Can you work these out from the model? Positions are in its coordinate system, mm. Face numbers are marked on the shaded views. A direction names the side the tool comes from. Coordinates: 2 decimals unless noted, no trailing zeros. Order: outer loops, then holes, each group sorted by start corner. A loop starts at its lowest first (then second) coordinate and runs counter-clockwise, first axis right, second up. Notation, with made-up numbers: M 30.5,9.25 L 52.5,9.25 A28 cw 52.5,44.25 Z; hole C 75,72 d2. An arc over 180 degrees is marked long. Answer as a JSON object with one key per item and string values.
from build123d import *
from build123d import SkipClean  # not in build123d's __all__

# Parameters (mm, degrees)
F1_DEPTH = 31.75
F2_DEPTH = 53.975
F3_DEPTH = 73.025
F0_W     = 31.75
F0_H     = 31.75
F4_DEPTH = 92.075
F5_DEPTH = 73.025


with BuildPart() as f1:
    # F0 (on Top) → F1 (new body)
    with BuildSketch(Plane.XY):
        Polygon((108.4912913322, 117.0880892358), (32.2912913322, 117.0880892358), (32.2912913322, 85.3380892358), (32.2912913322, 15.4880892358), (32.2912913322, -3.5619107642), (32.2912913322, -16.2619107642), (32.2912913322, -35.3119107642), (108.4912913322, -35.3119107642), (108.4912913322, 15.4880892358), (67.2162913322, 15.4880892358), (67.2162913322, 66.2880892358), (108.4912913322, 66.2880892358), align=None)
    extrude(amount=F1_DEPTH)



with BuildPart() as f2:
    # F0 (on Top) → F2 (new body)
    with BuildSketch(Plane.XY):
        with BuildLine():
            Line((0.5412913322, 117.0880892358), (-37.5587086678, 117.0880892358))
            Line((-37.5587086678, 117.0880892358), (-37.5587086678, 56.7630892358))
            ThreePointArc((-37.5587086678, 56.7630892358), (-21.6837086678, 40.8880892358), (-37.5587086678, 25.0130892358))
            Line((-37.5587086678, 25.0130892358), (-37.5587086678, -35.3119107642))
            Line((-37.5587086678, -35.3119107642), (0.5412913322, -35.3119107642))
            Line((0.5412913322, -35.3119107642), (0.5412913322, -3.5619107642))
            Line((0.5412913322, -3.5619107642), (0.5412913322, 15.4880892358))
            Line((0.5412913322, 15.4880892358), (0.5412913322, 85.3380892358))
            Line((0.5412913322, 85.3380892358), (0.5412913322, 117.0880892358))
        make_face()
    extrude(amount=F2_DEPTH)


with BuildPart() as f1_1:
    add(f1.part, clean=False)

    add(f2.part)  # F3 merges F2
    # F0 (on Top) → F3 (join)
    with BuildSketch(Plane.XY):
        Polygon((32.2912913322, 85.3380892358), (0.5412913322, 85.3380892358), (0.5412913322, 15.4880892358), (0.5412913322, -3.5619107642), (32.2912913322, -3.5619107642), (32.2912913322, 15.4880892358), align=None)
    extrude(amount=F3_DEPTH)

    # F0 (on Top) → F4 (join)
    with BuildSketch(Plane.XY):
        Polygon((32.2912913322, -3.5619107642), (0.5412913322, -3.5619107642), (0.5412913322, -35.3119107642), (32.2912913322, -35.3119107642), (32.2912913322, -16.2619107642), align=None)
        with Locations((16.4162913322, 101.2130892358)):
            Rectangle(F0_W, F0_H)
    extrude(amount=F4_DEPTH)

    # F0 (on Top) → F5 (join)
    with BuildSketch(Plane.XY):
        Polygon((32.2912913322, 85.3380892358), (0.5412913322, 85.3380892358), (0.5412913322, 15.4880892358), (0.5412913322, -3.5619107642), (32.2912913322, -3.5619107642), (32.2912913322, 15.4880892358), align=None)
    extrude(amount=F5_DEPTH)

    # F6: F1 across face


with BuildPart() as f1_2:
    add(f1_1.part, clean=False)
    with SkipClean():  # cleaning this boolean's faces spoils the solid; the shape is the same uncleaned
        add(f1_1.part.mirror(Plane(origin=(-37.5587086678, 86.9255892358, 26.9875), x_dir=(0, -1, 0), z_dir=(-1, 0, 0))), clean=False)


solid = f1_2.part
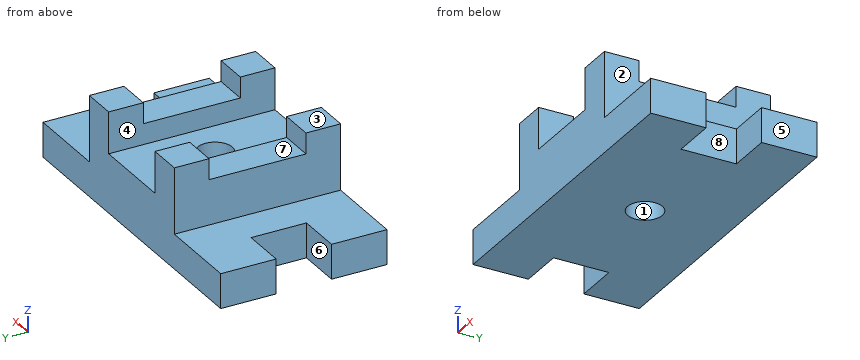
Item 1: I want a section at A-A, the plane x = 74. Write out the boundary of the cut face in (y, z), plus the area to 3 significant figures.
Answers follow:
{"outline": "M -35.31,0 L 15.49,0 L 15.49,31.75 L -35.31,31.75 Z; M 66.29,0 L 117.09,0 L 117.09,31.75 L 66.29,31.75 Z", "area": "3,230 mm^2"}
Item 2: I want a section at D-D, the plane x = 21. Write out the boundary of the cut face in (y, z) (3 decimals).
Answers follow:
{"outline": "M -35.312,0 L 117.088,0 L 117.088,92.075 L 85.338,92.075 L 85.338,73.025 L -3.562,73.025 L -3.562,92.075 L -35.312,92.075 Z"}
Item 3: Please list where these lines run through material, in increasing order: line 1 (X direction, y = -5, z = 70.5); line 2 (Y direction, x = 93, z = 12); line 3 (Y direction, x = -100, z = 74).
Answers follow:
{"line 1": "x = -107.41 to -75.66, 0.54 to 32.29", "line 2": "y = -35.31 to 15.49, 66.29 to 117.09", "line 3": "y = -35.31 to -3.56, 85.34 to 117.09"}
Item 4: If we mould it in two halves opening along X, with no side actions, what happens to the marked faces 1, 2 and 3? For each: pulls with the +X half, pulls with the -X half, needs draft (parallel to the pull), parting line crosses it, or undercut.
Answers follow:
{"face 1": "undercut", "face 2": "pulls with the +X half", "face 3": "needs draft"}
Item 5: Which directions (+Z, -Z, +X, -X, +Y, -Y) give clear straight access to the entire face, cutting with the end or side of a thin tool? Please do the marked faces 4, 5, 6, 7 and 8.
Answers follow:
{"face 4": "+Z, +Y, -Y", "face 5": "+Z, -Z, +X, +Y, -Y", "face 6": "+Z, -Z, -X", "face 7": "+Z, +X, -X", "face 8": "+Z, -Z, +X"}
Item 6: I want a section at C-C, the plane y = -7. Write out the boundary of the cut face in (x, z) (3 decimals), plus the area to 3 significant figures.
Answers follow:
{"outline": "M -183.609,0 L 108.491,0 L 108.491,31.75 L 32.291,31.75 L 32.291,92.075 L 0.541,92.075 L 0.541,53.975 L -75.659,53.975 L -75.659,92.075 L -107.409,92.075 L -107.409,31.75 L -183.609,31.75 Z", "area": "14,800 mm^2"}
Item 7: I'm going to push flat-ended pins straight in: pin 1 (19 mm diameter, centred on x = -37.56, y = 40.89, fed in from -Z); pin 2 (6 mm diameter, centred on y = 13, z = 57, fed in from +X); pin 3 (4 mm diameter, centred on x = -34, y = 9, fed in from -Z); pin 4 (12 mm diameter, centred on y = 55, z = 28.5, fed in from +X). Where does each tip first touch, or does it pass through?
Answers follow:
{"pin 1": "passes through", "pin 2": "stops at x = 32.29", "pin 3": "stops at z = 0", "pin 4": "stops at x = 67.22"}
Item 8: I want a section at B-B, the plane z = 69. Write out the boundary of the cut face in (x, y), plus the area to 3 significant figures.
Answers follow:
{"outline": "M -107.41,-35.31 L -75.66,-35.31 L -75.66,117.09 L -107.41,117.09 Z; M 0.54,-35.31 L 32.29,-35.31 L 32.29,117.09 L 0.54,117.09 Z", "area": "9,680 mm^2"}
